Check sheet for the modelled part. Datum: model origin and axes. Units: mm. A direction names the side the tool comes from. Give positions to 0.01 mm unless a question says otherwise; leave off trailing zeros. Loops run counter-clockwise (first coordinate to the right, second up) from the corner with the lowest first, then second, coordinate; pieces in that order, holes last. Notation, with made-up numbers: (3.5, 72.5) -> (62.5, 72.5) arc R28 cw to (62.5, 109.5) -> close; hole circle Ø8 at (-7.5, 50). An arc over 180 degrees is marked (long way). Write each question's results on one line, items separated by ' | '. Start each with the question number.
Item 1: Cross-section at A-A on z = -6. Enter the section's corners in (x, y), then the cut area to 3 significant figures.
Item 2: Access from +Z, -Z, +X, -X, +Y, -Y to the whole of each face (thin tool, end or side, straight path). Record for faces 1 (the face through (0, 0, 3)), 2 (the face through (0, 3, 13.499)), 3 (the face through (2.36, 2.54, -8.7)), 4 (the face through (-2.945, 2, 6)), 5 (the face through (3.055, 2, 7)).
Item 3: Cross-section at B-B on z = 11.75. Enter the section's corners in (x, y), then the cut area to 3 significant figures.
Item 4: Mould release check, pull along X, two halves, no side actions. Record for faces 6 (the face through (2.7, 2.5, 14.449)), 7 (the face through (3.555, 2, -5)), 8 (the face through (-3.445, 2, -5)), 9 (the face through (0, 2, -0.381)): pulls with the +X half, pulls with the -X half, needs draft (parallel to the pull), parting line crosses it, or undercut.
Item 5: Gauge pin test, flat ends, axial feed: pin 1 Ø3 at (y, z) = (3.5, -2.5) entering from +X; pin 2 Ø0.9 at (x, y) = (0, 2.5) entering from -Z; pin 3 Ø0.7 at (x, y) = (-2.5, 2) entering from -Z; pin 4 Ø1 at (x, z) = (-0.5, 1.5) entering from -Y. Record the tip position at first contact, or that the pin passes through.
Item 6: Scan lines: line 1 along X through (y, z) = (3.1, -7); line 2 along X through (y, z) = (3.1, 9.5); line 3 along Z through (x, y) = (1.25, 4.45). Record each from-to range of solid material in increasing order.
from build123d import *

# Parameters (mm, degrees)
BOSS_EXTRUDE1_DEPTH = 5
FILLET2_R           = 0.2
FILLET3_R           = 1
FILLET6_R           = 0.5
SKETCH3_W           = 7
SKETCH3_H           = 5
BOSS_EXTRUDE2_DEPTH = 7.2
SKETCH4_W           = 6
SKETCH4_H           = 5
BOSS_EXTRUDE3_DEPTH = 3.13
SKETCH5_W           = 5.25
SKETCH5_H           = 0.55
CUT_EXTRUDE1_DEPTH  = 6
FILLET8_R           = 0.25
SKETCH9_W           = 0.605295755
SKETCH9_H           = 5
CUT_EXTRUDE5_DEPTH  = 13
SKETCH10_W          = 0.5
SKETCH10_H          = 5
CUT_EXTRUDE6_DEPTH  = 13
FILLET16_R          = 0.25
SKETCH12_W          = 4
SKETCH12_H          = 5
CUT_EXTRUDE7_DEPTH  = 0.4
CUT_EXTRUDE8_DEPTH  = 0.5


with BuildPart() as part:
    # Sketch2 → Boss-Extrude1 (new body)
    with BuildSketch(Plane(origin=(0, 0, 0), x_dir=(1, 0, 0), z_dir=(0, 1, 0))):
        Polygon((-3.445470037, -4.119402442), (3.554529963, -4.119402442), (3.554529963, 8.054782302), (5.554529963, 8.054782302), (3.554529963, 8.982336318), (2.054529963, 8.982336318), (2.054529963, 0.380597558), (-1.945470037, 0.380597558), (-1.945470037, 8.982336318), (-3.445470037, 8.982336318), (-5.445470037, 8.054782302), (-3.445470037, 8.054782302), align=None)
    extrude(amount=BOSS_EXTRUDE1_DEPTH)

    # Fillet2
    fillet2_edges = [part.edges().sort_by_distance(p)[0] for p in [
        (-3.445470037, 2.5, -8.054782302),
        (3.554529963, 2.5, -8.054782302),
    ]]
    fillet(fillet2_edges, radius=FILLET2_R)

    # Fillet3
    fillet3_edges = [part.edges().sort_by_distance(p)[0] for p in [
        (-3.445470037, 2.5, -8.982336318),
        (-1.945470037, 2.5, -8.982336318),
        (2.054529963, 2.5, -8.982336318),
        (3.554529963, 2.5, -8.982336318),
    ]]
    fillet(fillet3_edges, radius=FILLET3_R)

    # Fillet6
    fillet6_edges = [part.edges().sort_by_distance(p)[0] for p in [
        (-1.945470037, 2.5, -0.380597558),
        (2.054529963, 2.5, -0.380597558),
    ]]
    fillet(fillet6_edges, radius=FILLET6_R)

    # Sketch3 → Boss-Extrude2 (add)
    with BuildSketch(Plane.XY.offset(4.119402442)):
        with Locations((0.054529963, 2.5)):
            Rectangle(SKETCH3_W, SKETCH3_H)
    extrude(amount=BOSS_EXTRUDE2_DEPTH)

    # Sketch4 → Boss-Extrude3 (add)
    with BuildSketch(Plane.XY.offset(11.319402442)):
        with Locations((0.054529963, 2.5)):
            Rectangle(SKETCH4_W, SKETCH4_H)
    extrude(amount=BOSS_EXTRUDE3_DEPTH)

    # Sketch5 → Cut-Extrude1 (cut)
    with BuildSketch(Plane(origin=(0, 5, 0), x_dir=(1, 0, 0), z_dir=(0, 1, 0))):
        with Locations((0.054529963, -13.774402442)):
            Rectangle(SKETCH5_W, SKETCH5_H)
    extrude(amount=-CUT_EXTRUDE1_DEPTH, mode=Mode.SUBTRACT)

    # Fillet8
    fillet8_edges = [part.edges().sort_by_distance(p)[0] for p in [
        (-5.445470037, 2.5, -8.054782302),
        (5.554529963, 2.5, -8.054782302),
    ]]
    fillet(fillet8_edges, radius=FILLET8_R)

    # Sketch9 → Cut-Extrude5 (cut)
    with BuildSketch(Plane.XY.offset(11.319402442)):
        with Locations((-3.248117915, 2.5)):
            Rectangle(SKETCH9_W, SKETCH9_H)
    extrude(amount=-CUT_EXTRUDE5_DEPTH, mode=Mode.SUBTRACT)

    # Sketch10 → Cut-Extrude6 (cut)
    with BuildSketch(Plane.XY.offset(11.319402442)):
        with Locations((3.304529963, 2.5)):
            Rectangle(SKETCH10_W, SKETCH10_H)
    extrude(amount=-CUT_EXTRUDE6_DEPTH, mode=Mode.SUBTRACT)

    # Fillet16
    fillet16_edges = [part.edges().sort_by_distance(p)[0] for p in [
        (-2.945470037, 2.5, -1.680597558),
        (3.054529963, 2.5, -1.680597558),
    ]]
    fillet(fillet16_edges, radius=FILLET16_R)

    # Sketch12 → Cut-Extrude7 (cut)
    with BuildSketch(Plane.XY.offset(14.449402442)):
        with Locations((0.054529963, 2.5)):
            Rectangle(SKETCH12_W, SKETCH12_H)
    extrude(amount=-CUT_EXTRUDE7_DEPTH, mode=Mode.SUBTRACT)

    # Sketch14 → Cut-Extrude8 (cut)
    with BuildSketch(Plane.XY.offset(14.449402442)):
        with BuildLine():
            Line((-1.945470037, 5), (-2.945470037, 5))
            ThreePointArc((-2.945470037, 5), (-2.204559454, 3.831888923), (-1.945470037, 2.473100986))
            Line((-1.945470037, 2.473100986), (-1.945470037, 5))
        make_face()
        with BuildLine():
            Line((-1.945470037, 0), (-1.945470037, 2.473100986))
            ThreePointArc((-1.945470037, 2.473100986), (-2.191277733, 1.14836624), (-2.895975223, 0))
            Line((-2.895975223, 0), (-1.945470037, 0))
        make_face()
        with BuildLine():
            Line((2.054529963, 0), (3.054529963, 0))
            ThreePointArc((3.054529963, 0), (2.313801958, 1.153708798), (2.054529963, 2.5))
            Line((2.054529963, 2.5), (2.054529963, 0))
        make_face()
        with BuildLine():
            ThreePointArc((2.054529963, 2.5), (2.313801958, 3.846291202), (3.054529963, 5))
            Line((3.054529963, 5), (2.054529963, 5))
            Line((2.054529963, 5), (2.054529963, 2.5))
        make_face()
    extrude(amount=-CUT_EXTRUDE8_DEPTH, mode=Mode.SUBTRACT)


solid = part.part
Answer sheet:
1) outline: (-3.45, 0) -> (-1.95, 0) -> (-1.95, 5) -> (-3.45, 5) -> close; (2.05, 0) -> (3.55, 0) -> (3.55, 5) -> (2.05, 5) -> close | area: 15.0 mm²
2) face 1: +Z, -Z, +X, -X, -Y | face 2: +Y, -Y | face 3: -Z, +Y, -Y | face 4: +Z, -X, +Y, -Y | face 5: +Z, +X, +Y, -Y
3) outline: (-2.95, 0) -> (3.05, 0) -> (3.05, 5) -> (-2.95, 5) -> close | area: 30.0 mm²
4) face 6: needs draft | face 7: pulls with the +X half | face 8: pulls with the -X half | face 9: undercut
5) pin 1: stops at x = 3.55 | pin 2: stops at z = -0.38 | pin 3: stops at z = -8.98 | pin 4: stops at y = 0
6) line 1: x = -3.45 to -1.95, 2.05 to 3.55 | line 2: x = -2.95 to 3.05 | line 3: z = -0.38 to 13.5
